Part model, mm, in its own coordinate system. A direction names the side the tool comes from. Give positions to 0.01 mm unless a question says otherwise; leave off trailing zeros. Order: outer loops, then holes, each group sorted by start corner. A loop starts at its lowest first (then second) coordinate and runs counter-clockwise, first axis right, second up. Notation, with made-up numbers: (48.25, 4.25) -> (57.25, 4.25) arc R20 ccw to (57.25, 42.25) -> close; hole circle Ø9 at (56, 39.25). An arc over 180 degrees is marked (long way). Write item = value, one per line. Start each with the question number.
Item 1: Band-saw the part on A-A on x = 17. Write the cut outline in (y, z), plus the area to 3 significant figures.
Item 2: Drill centre lines: line 1 along Z through (x, y) = (3, 35); line 2 along Y through (x, z) = (1.6, 0); line 3 along X through (y, z) = (2.35, 0). Where is each one in solid material? Low to high.
Item 3: Tool access for faces 5 (the face through (5.5, 28, 0)), 6 (the face through (3, 50, 0)): list every direction of +Z, -Z, +X, -X, +Y, -Y with a clear straight run to the whole face (end or side of a thin tool).
Item 4: Flat gauge pins, fed straight in: P1, Ø5, axis at x = 10.5, y = 8.5, coming from the -Z side (1 decimal); P2, Ø5, axis at x = 38, z = 1.5, coming from the +Y side; P3, Ø5, axis at y = 31, z = 2.5, coming from the +X side. Where does each tip first touch, or does it go through?
Item 5: Pull direction Z, two halves, no side cores. Call faces 1 (the face through (2.72, 19.44, -0.54)), 2 (the face through (2.72, 32.89, 1.34)), 3 (the face through (14, 5, 4.75)), 4 (the face through (50, 3, 0)): +Z half, -Z half, draft (parallel to the pull), parting line (faces both ways), or undercut.
Item 6: Band-saw the part on D-D on x = 23. Write the cut outline in (y, z).
Item 7: Band-saw the part on C-C on z = 0. Count the separate pieces of the cut face and the enclosed holes in it, plus the area to 3 significant figures.
```python
from build123d import *

# Parameters (mm, degrees)
EXTRUDE_1_DEPTH            = 4.75
HOLE_WIZARD_M61_AT_2_COUNT = 2
HOLE_WIZARD_M61_AT_2_PITCH = 18
CHAMFER_1_SIZE             = 0.5


with BuildPart() as part:
    # Эскиз1 → Бобышка-Вытянуть1 (new body, symmetric)
    with BuildSketch(Plane.XY):
        with BuildLine():
            Line((0, 50), (0, 7))
            ThreePointArc((0, 7), (2.050252532, 2.050252532), (7, 0))
            Line((7, 0), (50, 0))
            Line((50, 0), (50, 5.5))
            Line((50, 5.5), (7, 5.5))
            ThreePointArc((7, 5.5), (5.939339828, 5.939339828), (5.5, 7))
            Line((5.5, 7), (5.5, 50))
            Line((5.5, 50), (0, 50))
        make_face()
    extrude(amount=EXTRUDE_1_DEPTH, both=True)

    # Эскиз5 → Отверстие обработанное метчиком M61 (revolve, cut)
    with BuildSketch(Plane.ZX.offset(35)):
        Polygon((0, 0), (0, 5.5), (3.1, 5.5), (2.5, 4.9), (2.5, 0.6), (3.1, 0), align=None)
    hole_wizard_m61 = revolve(axis=Axis((-6.35, 35, 0), (1, 0, 0)), mode=Mode.SUBTRACT)

    # Отверстие обработанное метчиком M61 at 2: Отверстие обработанное метчиком M61 ×2
    with Locations(*[(0, -i * HOLE_WIZARD_M61_AT_2_PITCH, 0) for i in range(1, HOLE_WIZARD_M61_AT_2_COUNT)]):
        add(hole_wizard_m61, mode=Mode.SUBTRACT)

    # Зеркальное отражение1: Отверстие обработанное метчиком M61 across plane
    add(hole_wizard_m61.mirror(Plane(origin=(0, 0, 0), x_dir=(0, 0, 1), z_dir=(-0.707106781, 0.707106781, 0))), mode=Mode.SUBTRACT)

    # Зеркальное отражение1 copy 1 sketch → Зеркальное отражение1 copy 1 (revolve, cut)
    with BuildSketch(Plane(origin=(17, 0, 0), x_dir=(0, 0, 1), z_dir=(1, 0, 0))):
        Polygon((0, 0), (0, -5.5), (3.1, -5.5), (2.5, -4.9), (2.5, -0.6), (3.1, 0), align=None)
    revolve(axis=Axis((17, -6.35, 0), (0, -1, 0)), mode=Mode.SUBTRACT)

    # Фаска1
    chamfer_1_edges = [part.edges().sort_by_distance(p)[0] for p in [
        (2.75, 50, -4.75),
        (50, 2.75, 4.75),
        (2.75, 50, 4.75),
        (50, 2.75, -4.75),
    ]]
    chamfer(chamfer_1_edges, length=CHAMFER_1_SIZE)


solid = part.part
```
Values found:
q1.outline = (0, -4.75) -> (5.5, -4.75) -> (5.5, -3.1) -> (4.9, -2.5) -> (0.6, -2.5) -> (0, -3.1) -> close; (0, 3.1) -> (0.6, 2.5) -> (4.9, 2.5) -> (5.5, 3.1) -> (5.5, 4.75) -> (0, 4.75) -> close
q1.area = 24.0 mm^2
q2.line_1 = -4.75 to -2.5, 2.5 to 4.75
q2.line_2 = 2.55 to 14.5, 19.5 to 32.5, 37.5 to 50
q2.line_3 = 1.77 to 14.5, 19.5 to 32.5, 37.5 to 50
q3.face_5 = +Z, -Z, +X, +Y
q3.face_6 = +Z, -Z, +X, -X, +Y
q4.P1 = through
q4.P2 = 5.5
q4.P3 = 5.5
q5.face_1 = undercut
q5.face_2 = undercut
q5.face_3 = +Z half
q5.face_4 = draft
q6.outline = (0, -4.75) -> (5.5, -4.75) -> (5.5, 4.75) -> (0, 4.75) -> close
q7.separate_pieces = 5
q7.enclosed_holes = 0
q7.area = 397 mm^2
